Check sheet for the modelled part. Datum: model origin and axes. Units: mm. Coordinates: 2 decimals unless noted, no trailing zeros. Loops run counter-clockwise (first coordinate to the right, second up) from the corner with the lowest first, then second, coordinate; pieces in that order, holes last.
from build123d import *

# Parameters (mm, degrees)
F0_R     = 40
F1_DEPTH = 5
F3_D     = 5.5
F4_R     = 20
F5_DEPTH = 5.001
F6_SIZE  = 1


with BuildPart() as f1:
    # F0 (on Top) → F1 (new body)
    with BuildSketch(Plane.XY):
        Circle(F0_R)
    extrude(amount=F1_DEPTH)

    # F3 (through all)
    with Locations(Plane(origin=(0, 0, 0), x_dir=(1, 0, 0), z_dir=(0, 0, -1))):
        with Locations((0, 30), (25.980762, -15), (-25.980762, -15)):
            Hole(F3_D / 2)

    # F4 (on face) → F5 (cut, through all)
    with BuildSketch(Plane.XY.offset(5)):
        Circle(F4_R)
    extrude(amount=-F5_DEPTH, mode=Mode.SUBTRACT)

    # F6
    f6_edges = [f1.edges().sort_by_distance(p)[0] for p in [
        (-40, 0, 5),
        (-40, 0, 0),
        (-20, 0, 5),
        (-20, 0, 0),
    ]]
    chamfer(f6_edges, length=F6_SIZE)


solid = f1.part
(1) Section check C-C, the plane y = 15. Count the separate pieces of the cut face and the enclosed holes in it, plus the area to 3 significant figures.
(2) Section check A-A, the plane x = 0. Enter the section's corners in (y, z), plus the area to 4 significant figures.
(3) Draft check along X on faces 1 (the face through (-8.67, -39.05, 2.48)), 2 (the face through (17, -17, 0)), 3 (the face through (-4.336, -19.524, 2.521)), 4 (the face through (28.73, 14.88, 2.53)). Enter one of: pulls with the +X half, pulls with the -X half, needs draft (parallel to the pull), parting line crosses it, or undercut.
(4) Section check B-B, the plane y = 0. Enter the section's corners in (x, z).
(5) Gauge pin test, flat ends, axial feed: P1, Ø1.5, axis at x = 29, z = 3, coming from the +Y side; P2, Ø2, axis at y = 30, z = 2.5, coming from the -X side. Record the tip position at first contact, or that the pin passes through.
(6) Scan lines: line 1 along Y through (x, z) = (0, 2); line 2 along Y through (x, z) = (2.5, 4.8); line 3 along X through (y, z) = (0.5, 2.05). Record each from-to range of solid material in increasing order.
Determined:
1. separate pieces: 4
1. enclosed holes: 0
1. area: 178 mm2
2. outline: (-40, 1) - (-39, 0) - (-32.75, 0) - (-32.75, 5) - (-39, 5) - (-40, 4) - close; (-27.25, 0) - (-21, 0) - (-20, 1) - (-20, 4) - (-21, 5) - (-27.25, 5) - close; (20, 1) - (21, 0) - (39, 0) - (40, 1) - (40, 4) - (39, 5) - (21, 5) - (20, 4) - close
2. area: 168.5 mm2
3. face 1: parting line crosses it
3. face 2: needs draft
3. face 3: undercut
3. face 4: undercut
4. outline: (-40, 1) - (-39, 0) - (-21, 0) - (-20, 1) - (-20, 4) - (-21, 5) - (-39, 5) - (-40, 4) - close; (20, 1) - (21, 0) - (39, 0) - (40, 1) - (40, 4) - (39, 5) - (21, 5) - (20, 4) - close
5. P1: stops at y = 28.32
5. P2: stops at x = -27.55
6. line 1: y = -40 to -32.75, -27.25 to -20, 20 to 40
6. line 2: y = -39.12 to -31.15, -28.85 to -20.65, 20.65 to 39.12
6. line 3: x = -40 to -19.99, 19.99 to 40
